The listing builds one solid part. Answer for the finished solid, in the listing's coordinates (mm). A direction names the side the tool comes from. Round coordinates to 2 decimals unless told otherwise and drop trailing zeros. Write each loop counter-clockwise with the first axis right and the second up, starting at its lowest first coordinate (ties: lowest second). Pieces come first, ordered by that corner, then holes. Notation, with made-up numbers: (26, -5) - (40, -5) arc R15 ccw to (40, 13) - close; hole circle Ø3 at (6.5, 64). An arc over 180 degrees is marked (long way). Return JSON: item names as keys, results as strings. Group by question number.
(1) Section A-A, the plane x = -135 is taken. Write down the section's boundary in (y, z), then the cut area to 3 significant figures.
(2) Find the intervals of material crossed by line 1 along X through (y, z) = (-0.7, 15); line 2 along Z through (x, y) = (-196, -25.5); line 3 along Y through (x, z) = (36, 18), in increasing order. Write a range as [from, to].
(3) Which of the six approach directions +Z, -Z, +X, -X, +Y, -Y give full straight-line access (tool end or side, diameter ignored) to faces 5 (the cylindrical face through (52.998, -0.493, -0.176)), 6 (the flat face through (-182, -15, 30.737)), 7 (the flat face through (100.6, -0.49, -17.76))?
(4) Section C-C, the plane z = -4 is taken. Write down the section's boundary in (x, y).
(5) Section B-B, the plane y = -5.75 is taken. Write down the section's boundary in (x, z).
(6) Determine the mould class of faces 1 (the flat face through (-56.114, -0.493, -30.586)), 2 (the cylindrical face through (-220.068, -0.493, 13.959)), 3 (the flat face through (-182, -14, 31.737)), 4 (the cylindrical face through (-88.33, -12.86, 31.24)) for opening direction Z: +Z half, -Z half, draft (parallel to the pull), parting line (faces both ways), or undercut.
(7) Section D-D, the plane x = 67 is taken. Write down the section's boundary in (y, z), then the cut area to 3 significant figures.
(8) Each of these flat-tipped pins is pushed along its axis until it touches: pin 1 (12.5 mm diameter, centred on x = -185.5, y = -15.5, fed in from -Z); pin 2 (1.9 mm diameter, centred on y = -14, z = 31, fed in from -X); pin 3 (1.9 mm diameter, centred on y = -9, z = 31, fed in from +X); pin 4 (9.5 mm diameter, centred on x = -228, z = 15, fed in from +Y). Where does it stop, or does it pass through?
```python
from build123d import *

# Parameters (mm, degrees)
SKETCH2_R          = 8
BASE_FLANGE1_DEPTH = 1
EDGE_FLANGE5_DEPTH = 25
EDGE_FLANGE6_DEPTH = 25
EDGE_FLANGE7_DEPTH = 25
SKETCH29_R         = 3.25
CUT_EXTRUDE2_DEPTH = 10


# Sheet-metal steps are written as plain solids
with BuildPart() as part:
    # Sketch2 → Base-Flange1 (new body)
    with BuildSketch(Plane(origin=(0, 0, 0), x_dir=(1, 0, 0), z_dir=(0, 1, 0))):
        with BuildLine():
            Line((-41.298383568, 48.634081388), (76.701616432, 48.634081388))
            ThreePointArc((76.701616432, 48.634081388), (81.664016801, 47.315935025), (85.318183171, 43.708997903))
            Line((85.318183171, 43.708997903), (116.318183171, -8.925083485))
            ThreePointArc((116.318183171, -8.925083485), (117.349560964, -11.369949372), (117.701616432, -14))
            Line((117.701616432, -14), (117.701616432, -30))
            Line((117.701616432, -30), (-228, -30))
            ThreePointArc((-228, -30), (-242.841901676, -17.172085321), (-232.298383568, -0.629060619))
            Line((-232.298383568, -0.629060619), (-198.163972613, 9.580626254))
            ThreePointArc((-198.163972613, 9.580626254), (-196.746440448, 9.894601117), (-195.298383568, 10))
            Line((-195.298383568, 10), (-75.298383568, 10))
            ThreePointArc((-75.298383568, 10), (-67.251296492, 12.341232699), (-61.716223201, 18.634081388))
            Line((-61.716223201, 18.634081388), (-50.353157146, 42.878027129))
            ThreePointArc((-50.353157146, 42.878027129), (-46.663108285, 47.073259589), (-41.298383568, 48.634081388))
        make_face()
        with Locations(Location((-228, -15, 0), (0, 0, 270))):
            Circle(SKETCH2_R, mode=Mode.SUBTRACT)
        with BuildLine():
            Line((0, 8), (45, 8))
            ThreePointArc((45, 8), (53, 0), (45, -8))
            Line((45, -8), (0, -8))
            ThreePointArc((0, -8), (-8, 0), (0, 8))
        make_face(mode=Mode.SUBTRACT)
    extrude(amount=-BASE_FLANGE1_DEPTH)

    # Edge-Flange5 section (across the edge) → Edge-Flange5 (add)
    with BuildSketch(Plane(origin=(-172.5, -1, 30.7366), x_dir=(0, 0, -1), z_dir=(-1, 0, 0))):
        with BuildLine():
            Line((-1, 0.7366), (-1, 26))
            Line((-1, 26), (0, 26))
            Line((0, 26), (0, 0.7366))
            ThreePointArc((0, 0.7366), (0.215745145, 0.215745145), (0.7366, 0))
            Line((0.7366, 0), (0.7366, -1))
            ThreePointArc((0.7366, -1), (-0.491361636, -0.491361636), (-1, 0.7366))
        make_face()
    extrude(amount=EDGE_FLANGE5_DEPTH)

    # Edge-Flange6 section (across the edge) → Edge-Flange6 (add)
    with BuildSketch(Plane(origin=(-122.5, -1, 30.7366), x_dir=(0, 0, -1), z_dir=(-1, 0, 0))):
        with BuildLine():
            Line((-1, 0.7366), (-1, 26))
            Line((-1, 26), (0, 26))
            Line((0, 26), (0, 0.7366))
            ThreePointArc((0, 0.7366), (0.215745145, 0.215745145), (0.7366, 0))
            Line((0.7366, 0), (0.7366, -1))
            ThreePointArc((0.7366, -1), (-0.491361636, -0.491361636), (-1, 0.7366))
        make_face()
    extrude(amount=EDGE_FLANGE6_DEPTH)

    # Edge-Flange7 section (across the edge) → Edge-Flange7 (add)
    with BuildSketch(Plane(origin=(-72.5, -1, 30.7366), x_dir=(0, 0, -1), z_dir=(-1, 0, 0))):
        with BuildLine():
            Line((-1, 0.7366), (-1, 26))
            Line((-1, 26), (0, 26))
            Line((0, 26), (0, 0.7366))
            ThreePointArc((0, 0.7366), (0.215745145, 0.215745145), (0.7366, 0))
            Line((0.7366, 0), (0.7366, -1))
            ThreePointArc((0.7366, -1), (-0.491361636, -0.491361636), (-1, 0.7366))
        make_face()
    extrude(amount=EDGE_FLANGE7_DEPTH)

    # Sketch29 → Cut-Extrude2 (cut)
    with BuildSketch(Plane.XY.offset(31.7366)):
        with Locations((-85.082297009, -13)):
            Circle(SKETCH29_R)
        with Locations((-135, -14)):
            Circle(SKETCH29_R)
        with Locations((-185.477801268, -14.7366)):
            Circle(SKETCH29_R)
    extrude(amount=-CUT_EXTRUDE2_DEPTH, mode=Mode.SUBTRACT)


solid = part.part
```
Working result:
{
 "1": {"outline": "(-27, 30.74) - (-17.25, 30.74) - (-17.25, 31.74) - (-27, 31.74) - close; (-10.75, 30.74) - (-1.74, 30.74) arc R0.74 cw to (-1, 30) - (-1, -10) - (0, -10) - (0, 30) arc R1.74 ccw to (-1.74, 31.74) - (-10.75, 31.74) - close", "area": "60.7 mm^2"},
 "2": {"line 1": "x = [-243, -236], [-220, 117.7]", "line 2": "z = [30.74, 31.74]", "line 3": "y = [-1, 0]"},
 "3": {"face 5": "+Y, -Y", "face 6": "-Z, +X, -X, -Y", "face 7": "-Z, +X, +Y, -Y"},
 "4": {"outline": "(-216.82, -1) - (-6.93, -1) - (-6.93, 0) - (-216.82, 0) - close; (51.93, -1) - (108.71, -1) - (108.71, 0) - (51.93, 0) - close"},
 "5": {"outline": "(-197.5, 30.74) - (-172.5, 30.74) - (-172.5, 31.74) - (-197.5, 31.74) - close; (-147.5, 30.74) - (-122.5, 30.74) - (-122.5, 31.74) - (-147.5, 31.74) - close; (-97.5, 30.74) - (-72.5, 30.74) - (-72.5, 31.74) - (-97.5, 31.74) - close"},
 "6": {"face 1": "-Z half", "face 2": "undercut", "face 3": "+Z half", "face 4": "draft"},
 "7": {"outline": "(-1, -48.63) - (0, -48.63) - (0, 30) - (-1, 30) - close", "area": "78.6 mm^2"},
 "8": {"pin 1": "stops at z = 30.74", "pin 2": "stops at x = -197.5", "pin 3": "stops at x = -72.5", "pin 4": "passes through"}
}
